Autodesk Inventor part; units mm, degrees
ref_plane "YZ Plane" through (0, 0, 0) normal (1, 0, 0) x (0, 1, 0)
ref_plane "XZ Plane" through (0, 0, 0) normal (0, 1, 0) x (-1, 0, 0)
ref_plane "XY Plane" through (0, 0, 0) normal (0, 0, 1) x (1, 0, 0)
sketch "Sketch1" plane through (0, 0, 0) normal (0, 1, 0) x (-1, 0, 0)
  point P0 (0, 0)
sketch "Sketch2" plane through (0, 0, 0) normal (0, 1, 0) x (-1, 0, 0)
  line L0 (0, 0) -> (-38.1, 0)
  line L1 (-38.1, 0) -> (-38.1, -21.082)
  line L2 (-38.1, -21.082) -> (0, -21.082)
  line L3 (0, -21.082) -> (0, 0)
  dimension "d0" = 38.1
  dimension "d1" = 21.082
extrude "Extrusion1" add sketch "Sketch2" along normal blind 2.54
sketch "Sketch3" plane through (0, 2.54, 0) normal (0, 1, 0) x (1, 0, 0)
  line L0 (0, 0) -> (5.08, 0)
  line L1 (5.08, 0) -> (5.08, 5.08)
  line L2 (5.08, 5.08) -> (0, 5.08)
  line L3 (0, 5.08) -> (0, 0)
  line L4 (38.1, 0) -> (38.1, 21.082)
  line L5 (38.1, 21.082) -> (33.02, 21.082)
  line L6 (33.02, 21.082) -> (33.02, 16.002)
  line L7 (33.02, 16.002) -> (38.1, 16.002)
  line L8 (38.1, 16.002) -> (38.1, 21.082)
  line L9 (5.08, 5.08) -> (33.02, 5.08)
  line L10 (33.02, 5.08) -> (33.02, 16.002)
  line L11 (33.02, 16.002) -> (5.08, 16.002)
  line L12 (5.08, 16.002) -> (5.08, 5.08)
  dimension "d4" = 5.08
  dimension "d5" = 5.08
  dimension "d6" = 5.08
  dimension "d7" = 5.08
extrude "Extrusion2" cut sketch "Sketch3" against normal blind 2.54 contours L12 L11 L10 L9
sketch "Sketch4" plane through (0, 2.54, 0) normal (0, 1, 0) x (1, 0, 0)
  line L0 (0, 0) -> (38.1, 0)
  line L1 (0, 0) -> (10.16, 0)
  line L2 (10.16, 0) -> (10.16, 2.54)
  line L3 (10.16, 2.54) -> (0, 2.54)
  line L4 (0, 2.54) -> (0, 0)
  line L5 (38.1, 0) -> (27.94, 0)
  line L6 (27.94, 0) -> (27.94, 2.54)
  line L7 (27.94, 2.54) -> (38.1, 2.54)
  line L8 (38.1, 2.54) -> (38.1, 0)
  dimension "d10" = 10.16
  dimension "d11" = 2.54
  dimension "d12" = 10.16
  dimension "d13" = 2.54
extrude "Extrusion3" add sketch "Sketch4" along normal blind 20.32
sketch "Sketch5" plane through (10.16, 2.54, -2.54) normal (0, 0, -1) x (-1, 0, 0)
  line L0 (10.16, 20.32) -> (0, 20.32)
  line L1 (5.08, 20.32) -> (5.08, 10.16)
  point P0 (10.16, -2.54)
  dimension "d16" = 10.16
hole "Hole1" at (5.08, 12.7, -2.54) direction (0, 0, 1) diameter 5.08 end through all
sketch "Sketch6" plane through (38.1, 2.54, -2.54) normal (0, 0, -1) x (-1, 0, 0)
  line L0 (10.16, 20.32) -> (0, 20.32)
  line L1 (5.08, 20.32) -> (5.08, 10.16)
  point P0 (38.1, -2.54)
  dimension "d24" = 10.16
hole "Hole2" at (33.02, 12.7, -2.54) direction (0, 0, 1) diameter 5.08 end through all
properties part number "Actobotics Power Switch Mount"
Input: part model. Units: mm. Frame: model coordinates. A direction names the side the tool comes from. Coordinates: 2 decimals unless noted, no trailing zeros. Order: outer loops, then holes, each group sorted by start corner. A loop starts at its lowest first (then second) coordinate and runs counter-clockwise, first axis right, second up. Notation, with made-up numbers: M 50.5,85 L 88.5,85 A22 ccw 88.5,92 Z; hole C 2,22 d3. An arc over 180 degrees is marked long. Answer in a Markdown table with one row per item.
(1) Contact query for flat-ended pins moving along their axis: pin 1 Ø5 at (x, y) = (25.5, 15.5) entering from -Z; pin 2 Ø8 at (y, z) = (10, -5) entering from +X. Output: stop coordinate, or through.
Numbers:
| item | result |
|---|---|
| pin 1 | stops at z = -2.54 |
| pin 2 | stops at x = 38.1 |
(2) Section query C-C, the plane x = 6. Output: boundary loops of the cut face in (y, z).
Numbers:
| item | result |
|---|---|
| outline | M 0,-21.08 L 2.54,-21.08 L 2.54,-16 L 0,-16 Z; M 0,-5.08 L 2.54,-5.08 L 2.54,-2.54 L 10.33,-2.54 L 10.33,0 L 0,0 Z; M 15.07,-2.54 L 22.86,-2.54 L 22.86,0 L 15.07,0 Z |
(3) Access query for faces 4 (the flat face through (19, 1, -5.08)), 5 (the flat face through (10.16, 13, -1)), 6 (the flat face through (32, 10, -2.54)), 7 (the flat face through (0, 7, -2)), 8 (the cylindrical face through (3.36, 10.83, -1.25)). Directions: +Z, -Z, +X, -X, +Y, -Y. A direction counts if a zero-diameter tool reaches every point of the face in a straight line with its end or side. Return the directions, or none.
Numbers:
| item | result |
|---|---|
| face 4 | +Y, -Y |
| face 5 | +Z, -Z, +Y |
| face 6 | -Z, +X, -X, +Y |
| face 7 | +Z, -Z, -X, +Y, -Y |
| face 8 | +Z, -Z |
(4) Section query A-A, the plane y = 7.5. Output: boundary loops of the cut face in (x, z).
Numbers:
| item | result |
|---|---|
| outline | M 0,-2.54 L 10.16,-2.54 L 10.16,0 L 0,0 Z; M 27.94,-2.54 L 38.1,-2.54 L 38.1,0 L 27.94,0 Z |
(5) Section query D-D, the plane y = 12.7. Output: boundary loops of the cut face in (x, z).
Numbers:
| item | result |
|---|---|
| outline | M 0,-2.54 L 2.54,-2.54 L 2.54,0 L 0,0 Z; M 7.62,-2.54 L 10.16,-2.54 L 10.16,0 L 7.62,0 Z; M 27.94,-2.54 L 30.48,-2.54 L 30.48,0 L 27.94,0 Z; M 35.56,-2.54 L 38.1,-2.54 L 38.1,0 L 35.56,0 Z |
(6) Draft query along Z for faces 1 (the flat face through (27.94, 13, -1)), 2 (the flat face through (19, 1, -16.002)), 3 (the flat face through (19, 1, 0)). Return one class per face: pulls with the +Z half, pulls with the -Z half, needs draft (parallel to the pull), parting line crosses it, or undercut.
Numbers:
| item | result |
|---|---|
| face 1 | needs draft |
| face 2 | undercut |
| face 3 | pulls with the +Z half |
(7) Material intervals for line 1 (X direction, y = 12.7, z = -1.5); line 2 (Y direction, x = 33.02, z = -0.7); line 3 (Y direction, x = 6, z = -16.5), sorted ascending. Write a range as [from, to].
Numbers:
| item | result |
|---|---|
| line 1 | x = [0, 2.54], [7.62, 10.16], [27.94, 30.48], [35.56, 38.1] |
| line 2 | y = [0, 10.16], [15.24, 22.86] |
| line 3 | y = [0, 2.54] |
(8) Section query B-B, the plane x = 27.5. Output: boundary loops of the cut face in (y, z).
Numbers:
| item | result |
|---|---|
| outline | M 0,-21.08 L 2.54,-21.08 L 2.54,-16 L 0,-16 Z; M 0,-5.08 L 2.54,-5.08 L 2.54,0 L 0,0 Z |
